The listing builds one solid part. Answer for the finished solid, in the listing's coordinates (mm). Face numbers are marked on the shaded views. Coordinates: 2 decimals unless noted, no trailing zeros. Write each loop counter-clockwise with the first axis right and the second up, starting at its lowest first coordinate (ties: lowest second). Pieces come first, ordered by that corner, then holes.
from build123d import *

# Parameters (mm, degrees)
SKETCH1_R                = 2
BOSS_EXTRUDE1_DEPTH      = 3
BOSS_EXTRUDE3_DEPTH      = 3
SKETCH2_R                = 3.5
SKETCH2_R_2              = 2
BOSS_EXTRUDE2_DEPTH      = 3
SKETCH4_R                = 5
SKETCH4_R_2              = 1.65
BOSS_EXTRUDE4_DEPTH      = 6
FILLET1_R                = 10
SKETCH6_R                = 5
SKETCH6_R_2              = 1.65
BOSS_EXTRUDE5_DEPTH      = 6
FILLET2_R                = 10
CIRPATTERN4_COUNT        = 2
FILLET1_OF_CIRPATTERN4_R = 10
FILLET2_OF_MIRROR1_R     = 10
CHAMFER1_SIZE            = 0.5


with BuildPart() as part:
    # Sketch1 → Boss-Extrude1 (new body)
    with BuildSketch(Plane(origin=(0, 0, 0), x_dir=(1, 0, 0), z_dir=(0, 1, 0))):
        with BuildLine():
            Line((-39.5, -28), (39.5, -28))
            ThreePointArc((39.5, -28), (41.621320344, -27.121320344), (42.5, -25))
            Line((42.5, -25), (42.5, 25))
            ThreePointArc((42.5, 25), (41.621320344, 27.121320344), (39.5, 28))
            Line((39.5, 28), (-39.5, 28))
            ThreePointArc((-39.5, 28), (-41.621320344, 27.121320344), (-42.5, 25))
            Line((-42.5, 25), (-42.5, -25))
            ThreePointArc((-42.5, -25), (-41.621320344, -27.121320344), (-39.5, -28))
        make_face()
        with Locations(Location((-39, -24.5, 0), (0, 0, 270))):
            Circle(SKETCH1_R, mode=Mode.SUBTRACT)
        with Locations(Location((-39, 24.5, 0), (0, 0, 270))):
            Circle(SKETCH1_R, mode=Mode.SUBTRACT)
        with Locations(Location((19, 24.5, 0), (0, 0, 270))):
            Circle(SKETCH1_R, mode=Mode.SUBTRACT)
        with Locations(Location((19, -24.5, 0), (0, 0, 270))):
            Circle(SKETCH1_R, mode=Mode.SUBTRACT)
    extrude(amount=BOSS_EXTRUDE1_DEPTH)

    # Sketch3 → Boss-Extrude3 (add)
    with BuildSketch(Plane(origin=(0, 3, 0), x_dir=(1, 0, 0), z_dir=(0, 1, 0))):
        Polygon((-3, 3), (-72.5, 3), (-72.5, -3), (-3, -3), (-3, -72.5), (3, -72.5), (3, -3), (72.5, -3), (72.5, 3), (3, 3), (3, 72.5), (-3, 72.5), align=None)
    boss_extrude3 = extrude(amount=-BOSS_EXTRUDE3_DEPTH)

    # Sketch2 → Boss-Extrude2 (add)
    # profile 1 of 4: a face of its own
    with BuildSketch(Plane(origin=(0, 3, 0), x_dir=(1, 0, 0), z_dir=(0, 1, 0))):
        with Locations(Location((-39, -24.5, 0), (0, 0, 270))):
            Circle(SKETCH2_R)
        with Locations(Location((-39, -24.5, 0), (0, 0, 270))):
            Circle(SKETCH2_R_2, mode=Mode.SUBTRACT)
    # profile 2 of 4: a face of its own
    with BuildSketch(Plane(origin=(0, 3, 0), x_dir=(1, 0, 0), z_dir=(0, 1, 0))):
        with Locations(Location((-39, 24.5, 0), (0, 0, 90))):
            Circle(SKETCH2_R)
        with Locations(Location((-39, 24.5, 0), (0, 0, 270))):
            Circle(SKETCH2_R_2, mode=Mode.SUBTRACT)
    # profile 3 of 4: a face of its own
    with BuildSketch(Plane(origin=(0, 3, 0), x_dir=(1, 0, 0), z_dir=(0, 1, 0))):
        with Locations(Location((19, 24.5, 0), (0, 0, 90))):
            Circle(SKETCH2_R)
        with Locations(Location((19, 24.5, 0), (0, 0, 270))):
            Circle(SKETCH2_R_2, mode=Mode.SUBTRACT)
    # profile 4 of 4: a face of its own
    with BuildSketch(Plane(origin=(0, 3, 0), x_dir=(1, 0, 0), z_dir=(0, 1, 0))):
        with Locations(Location((19, -24.5, 0), (0, 0, 270))):
            Circle(SKETCH2_R)
        with Locations(Location((19, -24.5, 0), (0, 0, 270))):
            Circle(SKETCH2_R_2, mode=Mode.SUBTRACT)
    extrude(amount=BOSS_EXTRUDE2_DEPTH)

    # Sketch4 → Boss-Extrude4 (add)
    with BuildSketch(Plane.XY.offset(3)):
        with Locations((-72.5, 5)):
            Circle(SKETCH4_R)
        with Locations((-72.5, 5)):
            Circle(SKETCH4_R_2, mode=Mode.SUBTRACT)
    boss_extrude4 = extrude(amount=-BOSS_EXTRUDE4_DEPTH)

    # Fillet1
    fillet1_edges = [part.edges().sort_by_distance(p)[0] for p in [
        (-67.917424305, 3, 0),
    ]]
    fillet(fillet1_edges, radius=FILLET1_R)

    # Sketch6 → Boss-Extrude5 (add)
    with BuildSketch(Plane(origin=(3, 0, 0), x_dir=(0, 0, -1), z_dir=(1, 0, 0))):
        with Locations((-72.592807544, 4.999138602)):
            Circle(SKETCH6_R)
        with Locations((-72.592807544, 4.999138602)):
            Circle(SKETCH6_R_2, mode=Mode.SUBTRACT)
    boss_extrude5 = extrude(amount=-BOSS_EXTRUDE5_DEPTH)

    # Fillet2
    fillet2_edges = [part.edges().sort_by_distance(p)[0] for p in [
        (0, 3, 68.009856001),
    ]]
    fillet(fillet2_edges, radius=FILLET2_R)

    # CirPattern4: Boss-Extrude3, Boss-Extrude4 ×2 about axis
    cirpattern4_axis = Axis((0, 0, 0), (0, 1, 0))
    add([boss_extrude3.rotate(cirpattern4_axis, i * 360 / CIRPATTERN4_COUNT) for i in range(1, CIRPATTERN4_COUNT)])
    add([boss_extrude4.rotate(cirpattern4_axis, i * 360 / CIRPATTERN4_COUNT) for i in range(1, CIRPATTERN4_COUNT)])

    # Fillet1 of CirPattern4
    fillet1_of_cirpattern4_edges = [part.edges().sort_by_distance(p)[0] for p in [
        (67.917424305, 3, 0),
    ]]
    fillet(fillet1_of_cirpattern4_edges, radius=FILLET1_OF_CIRPATTERN4_R)

    # Mirror1: Boss-Extrude5 across plane
    add(boss_extrude5.mirror(Plane.XY))

    # Fillet2 of Mirror1
    fillet2_of_mirror1_edges = [part.edges().sort_by_distance(p)[0] for p in [
        (0, 3, -68.009856001),
    ]]
    fillet(fillet2_of_mirror1_edges, radius=FILLET2_OF_MIRROR1_R)

    # Chamfer1
    chamfer1_edges = [part.edges().sort_by_distance(p)[0] for p in [
        (-39, 6, 21),
        (-39, 6, -21),
        (19, 6, -21),
        (19, 6, 21),
    ]]
    chamfer(chamfer1_edges, length=CHAMFER1_SIZE)


solid = part.part
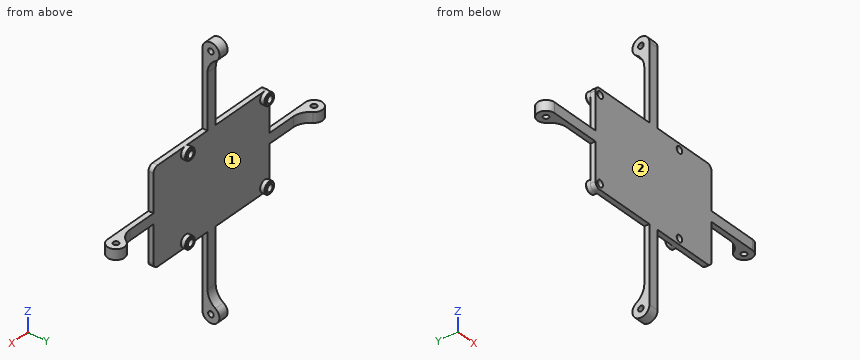
1. For a pull along Z with two mould halves and no side action, classify the marked faces 1 and 2 as pulls with the +Z half, pulls with the -Z half, needs draft (parallel to the pull), parting line crosses it, or undercut.
Results found:
face 1: undercut
face 2: needs draft
2. Section A-A on x = -54.5 is taken. Give the vertices of the cut face in (y, z), then the cut area to 3 significant figures.
Results found:
outline: (0, -3) - (3, -3) - (3, 3) - (0, 3) - close
area: 18.0 mm2
3. Flat-ended cylindrical pins translate along their axes: P1, Ø1.5, axis at x = 29, y = 2, coming from the -Z side; P2, Ø3, axis at x = 20, z = 23.5, coming from the +Y side; P3, Ø5, axis at x = 32.5, z = 20.5, coming from the -Y side; P4, Ø0.9, axis at x = -18, y = 1.5, coming from the +Z side. Find the tip coordinate at first contact, or state that the pin passes through.
Results found:
P1: stops at z = -28
P2: stops at y = 6
P3: stops at y = 0
P4: stops at z = 28
4. Find the intervals of material crossed by L1, parallel to Y at x = 25, z = 25.5; L2, parallel to Z at x = -67.5, y = 6; L3, parallel to Z at x = -19.5, y = 1, in increasing order.
Results found:
L1: y = 0 to 3
L2: z = -3 to 3
L3: z = -28 to 28
5. Section B-B on z = -38 is taken. Give the vertices of the cut face in (x, y), then the cut area to 3 significant figures.
Results found:
outline: (-3, 0) - (3, 0) - (3, 3) - (-3, 3) - close
area: 18.0 mm2
